Part model, mm, in its own coordinate system. A direction names the side the tool comes from. Round coordinates to 2 decimals unless told otherwise and drop trailing zeros. Write each loop counter-clockwise with the first axis right and the second up, starting at its lowest first coordinate (ties: lowest second). Pieces come first, ordered by that corner, then holes.
```python
from build123d import *

# Parameters (mm, degrees)
SKETCH1_W           = 10
SKETCH1_H           = 10
BOSS_EXTRUDE1_DEPTH = 3
SKETCH2_W           = 5
SKETCH2_H           = 5
BOSS_EXTRUDE2_DEPTH = 1
SKETCH3_R           = 1.85
CUT_EXTRUDE1_DEPTH  = 0.8
FILLET1_R           = 0.5
FILLET2_R           = 0.5


with BuildPart() as part:
    # Sketch1 → Boss-Extrude1 (new body)
    with BuildSketch(Plane.XY):
        Rectangle(SKETCH1_W, SKETCH1_H)
    extrude(amount=BOSS_EXTRUDE1_DEPTH)

    # Sketch2 → Boss-Extrude2 (add)
    with BuildSketch(Plane.XY.offset(3)):
        Rectangle(SKETCH2_W, SKETCH2_H)
    extrude(amount=BOSS_EXTRUDE2_DEPTH)

    # Sketch3 → Cut-Extrude1 (cut)
    with BuildSketch(Plane.XY.offset(4)):
        Circle(SKETCH3_R)
    extrude(amount=-CUT_EXTRUDE1_DEPTH, mode=Mode.SUBTRACT)

    # Fillet1
    fillet1_edges = [part.edges().sort_by_distance(p)[0] for p in [
        (5, -5, 1.5),
        (-5, -5, 1.5),
        (-5, 5, 1.5),
        (5, 5, 1.5),
    ]]
    fillet(fillet1_edges, radius=FILLET1_R)

    # Fillet2
    fillet2_edges = [part.edges().sort_by_distance(p)[0] for p in [
        (0, -5, 0),
        (5, 0, 0),
        (-5, 0, 0),
        (0, 5, 0),
        (4.853553391, -4.853553391, 0),
        (4.853553391, 4.853553391, 0),
        (-4.853553391, 4.853553391, 0),
        (-4.853553391, -4.853553391, 0),
    ]]
    fillet(fillet2_edges, radius=FILLET2_R)


solid = part.part
```
Q1. Mould opens along X. For faces 4 (the cylindrical face through (-0.401, -1.806, 3.606)), 5 (the flat face through (0, 0, 3.2)), 6 (the flat face through (0, -2.5, 3.5)), 7 (the flat face through (2.5, 0, 3.5)) say: +X half, -X half, draft (parallel to the pull), parting line (faces both ways), or undercut.
Values follow:
face 4: undercut
face 5: undercut
face 6: draft
face 7: +X half
Q2. Cut at A-A on z = 3.6. Write the cut outline in (x, y), plus the area to 3 significant figures.
Values follow:
outline: (-2.5, -2.5) - (2.5, -2.5) - (2.5, 2.5) - (-2.5, 2.5) - close; hole circle Ø3.7 at (0, 0)
area: 14.2 mm2
Q3. Drop a flat-ended pin along its axis: pin 1 (3 mm diameter, centred on x = 0, y = 0, fed in from +Z). Give the stop position or say it passes through.
Values follow:
pin 1: stops at z = 3.2
Q4. Wall check: L1, parallel to Y at x = 0, z = 3.45; L2, parallel to Z at x = 4.25, y = 1.5; L3, parallel to Y at x = 1, z = 3.4. Give the ranges that are in metal, low to high.
Values follow:
L1: y = -2.5 to -1.85, 1.85 to 2.5
L2: z = 0 to 3
L3: y = -2.5 to -1.56, 1.56 to 2.5
Q5. Cut at B-B on x = 0. Write the cut outline in (y, z), plus the area to 3 significant figures.
Values follow:
outline: (-5, 0.5) arc R0.5 ccw to (-4.5, 0) - (4.5, 0) arc R0.5 ccw to (5, 0.5) - (5, 3) - (2.5, 3) - (2.5, 4) - (1.85, 4) - (1.85, 3.2) - (-1.85, 3.2) - (-1.85, 4) - (-2.5, 4) - (-2.5, 3) - (-5, 3) - close
area: 31.9 mm2
Q6. Cut at C-C on y = 4. Write the cut outline in (x, z).
Values follow:
outline: (-5, 0.5) arc R0.5 ccw to (-4.5, 0) - (4.5, 0) arc R0.5 ccw to (5, 0.5) - (5, 3) - (-5, 3) - close
Q7. Which spindle directions (+Z, -Z, +X, -X, +Y, -Y) get a long thin tool onto all of the face, cutting with end or side? Do faces 1 (the flat face through (0, -5, 2)), 2 (the flat face through (-2.5, 0, 3.5)), 3 (the flat face through (0, 2.5, 3.5)). Say none if no direction does.
Values follow:
face 1: +Z, -Z, +X, -X, -Y
face 2: +Z, -X, +Y, -Y
face 3: +Z, +X, -X, +Y
